The listing builds one solid part. Answer for the finished solid, in the listing's coordinates (mm). A direction names the side the tool comes from. Coordinates: 2 decimals unless noted, no trailing zeros. Order: outer loops, then holes, each group sorted by start corner. A loop starts at its lowest first (then second) coordinate and runs counter-clockwise, first axis right, second up. Notation, with made-up numbers: (23, 31) - (82, 31) arc R32 cw to (82, 61) - close; hole circle Ø11 at (-8, -21.75). An arc over 180 degrees is marked (long way). Use one line per item in the form item = value. Start each with the question number.
Item 1: A tool of negligible diameter and unlimited length cuts with its end or side. For faces 4 (the flat face through (0, -128.889, 0)), 5 (the cylindrical face through (1.613, -141.359, -9.957)), 6 (the cylindrical face through (-6.05, -15.28, 1.9)), from which of +Z, -Z, +X, -X, +Y, -Y can it reach the whole face along a straight path? Write none if from no direction.
Item 2: The mould has two halves that part along X. Classify faces 1 (the cylindrical face through (-0.65, -12.93, -8.76)), 2 (the cylindrical face through (5.537, -75.867, -10.646)), 3 (the flat face through (5, 0, -5)): released by +X, released by -X, zero draft, split by the parting line, or undercut.
Item 3: Section A-A, the plane x = 0 is taken. Write down the section's boundary in (y, z), and give its area (3 significant figures).
Item 4: Each of these flat-tipped pins is pushed along its axis until it touches: pin 1 Ø7.5 at (x, z) = (0, 0) entering from -Y; pin 2 Ø8 at (x, y) = (0, -143.889) entering from +Z; pin 3 Ø1 at (y, z) = (-129, -5.5) entering from -X; pin 4 Ø8 at (x, y) = (-7.5, -84) entering from +Z. Where does it stop, or does it pass through?
Item 5: Section C-C, the plane z = 0 is taken. Write down the section's boundary in (x, y), and give its area (3 significant figures).
Item 6: Consider line 1 along Y through (x, z) = (0, -9); line 2 along Y through (x, z) = (2.5, 10.5); line 3 along Z through (x, y) = (0, -28). Determine where each line is inside the solid, lowest interval first. Write a range as [from, to].
Item 7: Section B-B, the plane y = -10 is taken. Write down the section's boundary in (x, z), and give its area (3 significant figures).
Item 8: Section D-D, the plane y = -131 is taken. Write down the section's boundary in (x, z), and give its area (3 significant figures).
from build123d import *

# Parameters (mm, degrees)
F0_R          = 12
F1_DEPTH      = 153.889
F2_R          = 8.50015
F3_DEPTH      = 25
F4_R          = 6.34015
F5_DEPTH      = 31
F6_R          = 3
F7_DEPTH      = 25
F7_DEPTH_BACK = 25


with BuildPart() as f1:
    # F0 (on Front) → F1 (new body)
    with BuildSketch(Plane.XZ):
        Circle(F0_R)
    extrude(amount=F1_DEPTH)

    # F2 (on face) → F3 (cut)
    with BuildSketch(Plane.XZ.offset(153.889)):
        Circle(F2_R)
    extrude(amount=-F3_DEPTH, mode=Mode.SUBTRACT)

    # F4 (on face) → F5 (cut)
    with BuildSketch(Plane(origin=(0, 0, 0), x_dir=(-1, 0, 0), z_dir=(0, 1, 0))):
        Circle(F4_R)
    extrude(amount=-F5_DEPTH, mode=Mode.SUBTRACT)

    # F6 (on Top) → F7 (cut, two sides)
    with BuildSketch(Plane.XY) as f7_sk:
        with Locations((0, -10)):
            Circle(F6_R)
        with Locations((0, -143.889)):
            Circle(F6_R)
    extrude(amount=-F7_DEPTH, mode=Mode.SUBTRACT)
    extrude(f7_sk.sketch, amount=F7_DEPTH_BACK, mode=Mode.SUBTRACT)


solid = f1.part
Response:
q1.face_4 = -Y
q1.face_5 = +Z, -Z
q1.face_6 = +Y
q2.face_1 = undercut
q2.face_2 = split by the parting line
q2.face_3 = zero draft
q3.outline = (-153.89, -12) - (-146.89, -12) - (-146.89, -8.5) - (-153.89, -8.5) - close; (-153.89, 8.5) - (-146.89, 8.5) - (-146.89, 12) - (-153.89, 12) - close; (-140.89, -12) - (-13, -12) - (-13, -6.34) - (-31, -6.34) - (-31, 6.34) - (-13, 6.34) - (-13, 12) - (-140.89, 12) - (-140.89, 8.5) - (-128.89, 8.5) - (-128.89, -8.5) - (-140.89, -8.5) - close; (-7, -12) - (0, -12) - (0, -6.34) - (-7, -6.34) - close; (-7, 6.34) - (0, 6.34) - (0, 12) - (-7, 12) - close
q3.area = 2,770 mm2
q4.pin_1 = -128.89
q4.pin_2 = 12
q4.pin_3 = -10.91
q4.pin_4 = 11.48
q5.outline = (-12, -153.89) - (-8.5, -153.89) - (-8.5, -128.89) - (8.5, -128.89) - (8.5, -153.89) - (12, -153.89) - (12, 0) - (6.34, 0) - (6.34, -31) - (-6.34, -31) - (-6.34, 0) - (-12, 0) - close
q5.area = 2,880 mm2
q6.line_1 = [-153.89, -146.89], [-140.89, -13], [-7, 0]
q6.line_2 = [-153.89, -145.55], [-142.23, -11.66], [-8.34, 0]
q6.line_3 = [-12, -6.34], [6.34, 12]
q7.outline = (-3, -11.62) - (-3, -5.59) arc R6.34 cw to (-3, 5.59) - (-3, 11.62) arc R12 ccw to start; (3, -11.62) arc R12 ccw to (3, 11.62) - (3, 5.59) arc R6.34 cw to (3, -5.59) - close
q7.area = 257 mm2
q8.outline = circle Ø24 at (0, 0); hole circle Ø17 at (0, 0)
q8.area = 225 mm2
